The listing builds one solid part. Answer for the finished solid, in the listing's coordinates (mm). A direction names the side the tool comes from. Round coordinates to 2 decimals unless told otherwise and drop trailing zeros. Order: outer loops, then holes, each group sorted by start corner. A loop starts at its lowest first (then second) coordinate and runs counter-clockwise, first axis right, second up. Notation, with made-up numbers: M 24,75.25 L 50,75.25 A13 cw 50,94.25 Z; hole C 0,85 d9. An arc over 180 degrees is marked long. Write item = value, one per line. Start each with the question number.
(1) A cutting plane is placed at A-A, the plane z = 4.05. Determine the outline of the cut face in (x, y), and give its area (3 significant figures).
(2) A cutting plane is placed at C-C, the plane x = 33.5. Determine the outline of the cut face in (y, z), and give its area (3 significant figures).
(3) Straight lines are drawn through the part: probe 1 along Z at (x, y) = (34.5, 7.5); probe 2 along Y at (x, z) = (53.5, 0.7); probe 3 along Y at (x, z) = (54, 4.45). For each, find the intervals that lie inside material, in ascending order. Write a range as from..to.
(4) For a pull along Y with two mould halves and no side action, classify faces 5 (the face through (45.5, 27, 1)), 6 (the face through (2.2, 71, 3)), 7 (the face through (4, 10, 3)) as released by +Y, released by -Y, zero draft, split by the parting line, or undercut.
(5) Which of the six approach directions +Z, -Z, +X, -X, +Y, -Y give full straight-line access (tool end or side, diameter ignored) to faces 1 (the face through (57.8, 71, 3)), 2 (the face through (48, 4, 3)), 3 (the face through (10, 4, 3)), 4 (the face through (15.5, 27, 1))?
(6) Each of these flat-tipped pins is pushed along its axis until it touches: pin 1 (10 mm diameter, centred on x = 50, y = 74.5, fed in from +Z); pin 2 (2 mm diameter, centred on x = 49, y = 3.5, fed in from +Z); pin 3 (1.5 mm diameter, centred on x = 3.5, z = 3, fed in from +Y); pin 4 (3 mm diameter, centred on y = 40.5, z = 5, fed in from -X). Where does it stop, or does it pass through?
(7) A cutting plane is placed at B-B, the plane y = 36.5. Determine the outline of the cut face in (x, z).
(8) A cutting plane is placed at D-D, the plane y = 89. Determine the outline of the cut face in (x, z).
from build123d import *

# Parameters (mm, degrees)
PAD_DEPTH     = 2
SKETCH002_W   = 2
SKETCH002_H   = 3
SKETCH002_W_2 = 3
SKETCH002_H_2 = 2
PAD001_DEPTH  = 3
SKETCH003_W   = 30
SKETCH003_H   = 5.833333
SKETCH003_H_2 = 5.833334
POCKET_DEPTH  = 5
SKETCH004_R   = 1.5
PAD002_DEPTH  = 4


with BuildPart() as part:
    # Sketch → Pad (new body)
    with BuildSketch(Plane.XY):
        with BuildLine():
            Line((60, 8), (60, 82.000001))
            ThreePointArc((60, 82.000001), (58.434586, 89.869877), (53.976662, 96.541638))
            Line((40.541631, 109.976664), (53.976662, 96.541638))
            ThreePointArc((40.541631, 109.976664), (33.869872, 114.434584), (25.999999, 115.999997))
            Line((7.999999, 115.999997), (25.999999, 115.999997))
            ThreePointArc((7.999999, 115.999997), (2.343146, 113.656851), (0, 107.999998))
            Line((0, 107.999998), (0, 8))
            ThreePointArc((0, 8), (2.343146, 2.343146), (8, 0))
            Line((8, 0), (52, 0))
            ThreePointArc((52, 0), (57.656854, 2.343146), (60, 8))
        make_face()
    extrude(amount=PAD_DEPTH)

    # Sketch002 → Pad001 (new body)
    with BuildSketch(Plane.XY.offset(2)):
        with Locations((11, 3.7)):
            Rectangle(SKETCH002_W, SKETCH002_H)
        with Locations((3.7, 11)):
            Rectangle(SKETCH002_W_2, SKETCH002_H_2)
        with Locations((49, 3.7)):
            Rectangle(SKETCH002_W, SKETCH002_H)
        with Locations((56.3, 11)):
            Rectangle(SKETCH002_W_2, SKETCH002_H_2)
        with Locations((56.3, 71)):
            Rectangle(SKETCH002_W_2, SKETCH002_H_2)
        with Locations((3.7, 71)):
            Rectangle(SKETCH002_W_2, SKETCH002_H_2)
    extrude(amount=PAD001_DEPTH)

    # Sketch003 → Pocket (cut)
    with BuildSketch(Plane.XY.offset(2)):
        with Locations((30.5, 66.083333)):
            Rectangle(SKETCH003_W, SKETCH003_H)
        with Locations((30.5, 56.25)):
            Rectangle(SKETCH003_W, SKETCH003_H_2)
        with Locations((30.5, 46.416666)):
            Rectangle(SKETCH003_W, SKETCH003_H)
        with Locations((30.5, 36.583333)):
            Rectangle(SKETCH003_W, SKETCH003_H)
        with Locations((30.5, 26.75)):
            Rectangle(SKETCH003_W, SKETCH003_H_2)
        with Locations((30.5, 16.916666)):
            Rectangle(SKETCH003_W, SKETCH003_H)
    extrude(amount=-POCKET_DEPTH, mode=Mode.SUBTRACT)

    # Sketch004 → Pad002 (new body)
    with BuildSketch(Plane.XY.offset(2)):
        with Locations((37.247765, 107.8)):
            Circle(SKETCH004_R)
        with Locations((54.5, 89)):
            Circle(SKETCH004_R)
    extrude(amount=PAD002_DEPTH)


solid = part.part
Reported:
q1.outline = M 2.2,10 L 5.2,10 L 5.2,12 L 2.2,12 Z; M 2.2,70 L 5.2,70 L 5.2,72 L 2.2,72 Z; M 10,2.2 L 12,2.2 L 12,5.2 L 10,5.2 Z; C 37.25,107.8 d3; M 48,2.2 L 50,2.2 L 50,5.2 L 48,5.2 Z; C 54.5,89 d3; M 54.8,10 L 57.8,10 L 57.8,12 L 54.8,12 Z; M 54.8,70 L 57.8,70 L 57.8,72 L 54.8,72 Z
q1.area = 50.1 mm²
q2.outline = M 0,0 L 14,0 L 14,2 L 0,2 Z; M 19.83,0 L 23.83,0 L 23.83,2 L 19.83,2 Z; M 29.67,0 L 33.67,0 L 33.67,2 L 29.67,2 Z; M 39.5,0 L 43.5,0 L 43.5,2 L 39.5,2 Z; M 49.33,0 L 53.33,0 L 53.33,2 L 49.33,2 Z; M 59.17,0 L 63.17,0 L 63.17,2 L 59.17,2 Z; M 69,0 L 114.58,0 L 114.58,2 L 69,2 Z
q2.area = 159 mm²
q3.probe_1 = 0..2
q3.probe_2 = 0.14..97.02
q3.probe_3 = 87.59..90.41
q4.face_5 = undercut
q4.face_6 = zero draft
q4.face_7 = released by -Y
q5.face_1 = +Z, +X, +Y, -Y
q5.face_2 = +Z, +Y, -Y
q5.face_3 = +Z, -X, +Y, -Y
q5.face_4 = +Z, -Z
q6.pin_1 = 2
q6.pin_2 = 5
q6.pin_3 = 72
q6.pin_4 = through
q7.outline = M 0,0 L 15.5,0 L 15.5,2 L 0,2 Z; M 45.5,0 L 60,0 L 60,2 L 45.5,2 Z
q8.outline = M 0,0 L 58.77,0 L 58.77,2 L 56,2 L 56,6 L 53,6 L 53,2 L 0,2 Z
